```python
from build123d import *

# Parameters (mm, degrees)
F1_DEPTH  = 900
F3_W      = 100
F3_H      = 100
F4_DEPTH  = 10
F6_W      = 100
F6_H      = 100
F7_DEPTH  = 10
F8_R      = 6
F9_DEPTH  = 10
F10_R     = 6
F11_DEPTH = 10


with BuildPart() as f1:
    # F0 (on Front) → F1 (new body)
    with BuildSketch(Plane.XZ):
        with BuildLine():
            ThreePointArc((50, 45), (48.535534, 48.535534), (45, 50))
            Line((45, 50), (-45, 50))
            ThreePointArc((-45, 50), (-48.535534, 48.535534), (-50, 45))
            Line((-50, 45), (-50, -45))
            ThreePointArc((-50, -45), (-48.535534, -48.535534), (-45, -50))
            Line((-45, -50), (45, -50))
            ThreePointArc((45, -50), (48.535534, -48.535534), (50, -45))
            Line((50, -45), (50, 45))
        make_face()
        with BuildLine():
            ThreePointArc((-47, 45), (-46.414214, 46.414214), (-45, 47))
            Line((-45, 47), (45, 47))
            ThreePointArc((45, 47), (46.414214, 46.414214), (47, 45))
            Line((47, 45), (47, -45))
            ThreePointArc((47, -45), (46.414214, -46.414214), (45, -47))
            Line((45, -47), (-45, -47))
            ThreePointArc((-45, -47), (-46.414214, -46.414214), (-47, -45))
            Line((-47, -45), (-47, 45))
        make_face(mode=Mode.SUBTRACT)
    extrude(amount=-F1_DEPTH)

    # F3 (on offset) → F4 (join)
    with BuildSketch(Plane.XZ):
        Rectangle(F3_W, F3_H)
    extrude(amount=-F4_DEPTH)

    # F6 (on offset) → F7 (join)
    with BuildSketch(Plane(origin=(0, 900, 0), x_dir=(1, 0, 0), z_dir=(0, 1, 0))):
        Rectangle(F6_W, F6_H)
    extrude(amount=-F7_DEPTH)

    # F8 (on face) → F9 (cut, through all)
    with BuildSketch(Plane(origin=(0, 900, 0), x_dir=(-1, 0, 0), z_dir=(0, 1, 0))):
        with Locations((-29, 29)):
            Circle(F8_R)
        with Locations((29, 29)):
            Circle(F8_R)
        with Locations((29, -29)):
            Circle(F8_R)
        with Locations((-29, -29)):
            Circle(F8_R)
    extrude(amount=-F9_DEPTH, mode=Mode.SUBTRACT)

    # F10 (on face) → F11 (cut, through all)
    with BuildSketch(Plane.XZ):
        with Locations((-29, 29)):
            Circle(F10_R)
        with Locations((29, 29)):
            Circle(F10_R)
        with Locations((29, -29)):
            Circle(F10_R)
        with Locations((-29, -29)):
            Circle(F10_R)
    extrude(amount=-F11_DEPTH, mode=Mode.SUBTRACT)


solid = f1.part
```
Input: part model. Units: mm. Frame: model coordinates. A direction names the side the tool comes from. Coordinates: 2 decimals unless noted, no trailing zeros. Write each loop counter-clockwise with the first axis right and the second up, starting at its lowest first coordinate (ties: lowest second). Pieces come first, ordered by that corner, then holes. Notation, with made-up numbers: (78.5, -23.5) -> (84.5, -23.5) arc R18 ccw to (84.5, 2.5) -> close; hole circle Ø5 at (30, 42). An arc over 180 degrees is marked (long way). Answer as a JSON object with one key per item and string values.
1. Section A-A on y = 577. Return the cut outline in (x, z), then the cut area to 3 significant figures.
Result set:
{"outline": "(-50, -45) arc R5 ccw to (-45, -50) -> (45, -50) arc R5 ccw to (50, -45) -> (50, 45) arc R5 ccw to (45, 50) -> (-45, 50) arc R5 ccw to (-50, 45) -> close; hole (-47, -45) arc R2 ccw to (-45, -47) -> (45, -47) arc R2 ccw to (47, -45) -> (47, 45) arc R2 ccw to (45, 47) -> (-45, 47) arc R2 ccw to (-47, 45) -> close", "area": "1,150 mm2"}
2. Section B-B on z = 2. Return the cut outline in (x, y), then the cut area to 3 significant figures.
Result set:
{"outline": "(-50, 0) -> (50, 0) -> (50, 900) -> (-50, 900) -> close; hole (-47, 10) -> (47, 10) -> (47, 890) -> (-47, 890) -> close", "area": "7,280 mm2"}
3. Mould query, pull axis Z, two halves, no side actions, for faces 1 (the face through (-1, 456, 50)), 2 (the face through (-50, 456, 1)), 3 (the face through (-47, 444, -1)). Classes: released by +Z, released by -Z, zero draft, split by the parting line, or undercut.
Result set:
{"face 1": "released by +Z", "face 2": "zero draft", "face 3": "undercut"}
4. Material intervals for line 1 (Z direction, x = -29, y = 7.75); line 2 (Z direction, x = 17, y = 506.5); line 3 (Z direction, x = -45.5, y = 827), sorted ascending. Write a range as from..to.
Result set:
{"line 1": "z = -50..-35, -23..23, 35..50", "line 2": "z = -50..-47, 47..50", "line 3": "z = -49.97..-46.94, 46.94..49.97"}
5. First-contact query: P1, Ø9.5, axis at x = 29, z = 29, coming from the +Y side. Flat tip, straight axial feed; report the tip coordinate or a pass-through.
Result set:
{"P1": "passes through"}
6. Section C-C on x = -4.5. Return the cut outline in (y, z), then the cut area to 3 significant figures.
Result set:
{"outline": "(0, -50) -> (900, -50) -> (900, 50) -> (0, 50) -> close; hole (10, -47) -> (890, -47) -> (890, 47) -> (10, 47) -> close", "area": "7,280 mm2"}
7. Access query for faces 4 (the face through (-1, 890, -1)), 5 (the face through (-1, 444, -50)). Directions: +Z, -Z, +X, -X, +Y, -Y. A direction counts if a zero-diameter tool reaches every point of the face in a straight line with its end or side. Return the directions, or none.
Result set:
{"face 4": "none", "face 5": "-Z, +X, -X, +Y, -Y"}
